Here's how the part is built. I have some questions about the finished solid (model axes, mm). A direction names the side the tool comes from. Round coordinates to 2 decimals unless told otherwise and drop trailing zeros. Loops run counter-clockwise (first coordinate to the right, second up) from the corner with the lowest first, then second, coordinate; pieces in that order, holes last. Notation, with made-up numbers: M 9,50 L 14,50 A29 ccw 14,88 Z; hole C 11.25,-22 d6. An arc over 180 degrees is marked long. Use a Markdown table: item, result.
from build123d import *

# Parameters (mm, degrees)
SKETCH1_W                    = 112.686822752
SKETCH1_H                    = 63.120861651
SKETCH1_R                    = 5.443424695
BASE_FLANGE1_DEPTH           = 0.7366
EDGE_FLANGE1_STRIP_W         = 4.4196
EDGE_FLANGE1_STRIP_H         = 0.7366
EDGE_FLANGE1_STRIP_CUT_DEPTH = 112.686822752
EDGE_FLANGE1_DEPTH           = 112.686822752
EDGE_FLANGE2_STRIP_W         = 4.4196
EDGE_FLANGE2_STRIP_H         = 0.7366
EDGE_FLANGE2_STRIP_CUT_DEPTH = 112.686822752
EDGE_FLANGE2_DEPTH           = 112.686822752


# Sheet-metal steps are written as plain solids
with BuildPart() as part:
    # Sketch1 → Base-Flange1 (new body)
    with BuildSketch(Plane(origin=(0, 0, 0), x_dir=(1, 0, 0), z_dir=(0, 1, 0))):
        with Locations((56.343411376, 31.560430826)):
            Rectangle(SKETCH1_W, SKETCH1_H)
        with Locations(Location((50.380635498, 49.990828995, 0), (0, 0, 270))):
            Circle(SKETCH1_R, mode=Mode.SUBTRACT)
        with Locations(Location((50.380635498, 13.130032656, 0), (0, 0, 90))):
            Circle(SKETCH1_R, mode=Mode.SUBTRACT)
    extrude(amount=-BASE_FLANGE1_DEPTH)

    # Edge-Flange1 strip (across the edge) → Edge-Flange1 strip cut (cut)
    with BuildSketch(Plane(origin=(112.686822752, 0, -63.120861651), x_dir=(0, 0, 1), z_dir=(-1, 0, 0))):
        with Locations((-0.7366, -0.3683)):
            Rectangle(EDGE_FLANGE1_STRIP_W, EDGE_FLANGE1_STRIP_H)
    extrude(amount=EDGE_FLANGE1_STRIP_CUT_DEPTH, mode=Mode.SUBTRACT)

    # Edge-Flange1 section (across the edge) → Edge-Flange1 (add)
    with BuildSketch(Plane(origin=(112.686822752, 0, -63.120861651), x_dir=(0, 0, 1), z_dir=(-1, 0, 0))):
        with BuildLine():
            Line((0, 0.7366), (0, 3.2634))
            Line((0, 3.2634), (0.7366, 3.2634))
            Line((0.7366, 3.2634), (0.7366, 0.7366))
            ThreePointArc((0.7366, 0.7366), (0.952345145, 0.215745145), (1.4732, 0))
            Line((1.4732, 0), (1.4732, -0.7366))
            ThreePointArc((1.4732, -0.7366), (0.43149029, -0.30510971), (0, 0.7366))
        make_face()
    extrude(amount=EDGE_FLANGE1_DEPTH)

    # Edge-Flange2 strip (across the edge) → Edge-Flange2 strip cut (cut)
    with BuildSketch(Plane(origin=(112.686822752, 3.2634, -62.384261651), x_dir=(0, -1, 0), z_dir=(-1, 0, 0))):
        with Locations((-0.7366, -0.3683)):
            Rectangle(EDGE_FLANGE2_STRIP_W, EDGE_FLANGE2_STRIP_H)
    extrude(amount=EDGE_FLANGE2_STRIP_CUT_DEPTH, mode=Mode.SUBTRACT)

    # Edge-Flange2 section (across the edge) → Edge-Flange2 (add)
    with BuildSketch(Plane(origin=(112.686822752, 3.2634, -62.384261651), x_dir=(0, -1, 0), z_dir=(-1, 0, 0))):
        with BuildLine():
            Line((0, 0.7366), (0, 61.2634))
            Line((0, 61.2634), (0.7366, 61.2634))
            Line((0.7366, 61.2634), (0.7366, 0.7366))
            ThreePointArc((0.7366, 0.7366), (0.952345145, 0.215745145), (1.4732, 0))
            Line((1.4732, 0), (1.4732, -0.7366))
            ThreePointArc((1.4732, -0.7366), (0.43149029, -0.30510971), (0, 0.7366))
        make_face()
    extrude(amount=EDGE_FLANGE2_DEPTH)


solid = part.part
1. I need wall thicknesses on probe 1 along Y at (x, z) = (16, -15); probe 2 along X at (y, z) = (-0.4, -48); probe 3 along Z at (x, y) = (94.5, 3.05). Which ranges of each line are inside material? Lowest first, please. Write a range as from..to.
Answer sheet:
| item | result |
|---|---|
| probe 1 | -0.74..0, 2.53..3.26 |
| probe 2 | 0..45.31, 55.45..112.69 |
| probe 3 | -62.41..-1.12 |
2. We'd pull the mould along Z, two halves only. Please class faces 1 (the face through (57, 2.527, -31)), 2 (the face through (52.02, -0.36, -44.8)): +Z half, -Z half, draft (parallel to the pull), parting line (faces both ways), or undercut.
Answer sheet:
| item | result |
|---|---|
| face 1 | draft |
| face 2 | undercut |
3. Imagine slicing it at C-C, the plane z = -48.5. Write out the boundary of the cut face in (x, y).
Answer sheet:
| item | result |
|---|---|
| outline | M 0,-0.74 L 45.15,-0.74 L 45.15,0 L 0,0 Z; M 0,2.53 L 112.69,2.53 L 112.69,3.26 L 0,3.26 Z; M 55.62,-0.74 L 112.69,-0.74 L 112.69,0 L 55.62,0 Z |
4. Imagine slicing it at B-B, the plane x = 104. Write out the boundary of the cut face in (y, z), then the cut area to 3 significant figures.
Answer sheet:
| item | result |
|---|---|
| outline | M -0.74,-61.65 A1.47 ccw 0.74,-63.12 L 1.79,-63.12 A1.47 ccw 3.26,-61.65 L 3.26,-1.12 L 2.53,-1.12 L 2.53,-61.65 A0.74 cw 1.79,-62.38 L 0.74,-62.38 A0.74 cw 0,-61.65 L 0,0 L -0.74,0 Z |
| area | 93.3 mm2 |
5. For pin 1 Ø1.5 at (x, y) = (39, 2.5) entering from +Z; pin 2 Ø1.2 at (x, y) = (78, 1.5) entering from +Z; pin 3 Ø17.5 at (x, z) = (50.38, -13.13) entering from -Y, each with a flat end and sliding along its axis, tell me the tip position at first contact or that it passes through.
Answer sheet:
| item | result |
|---|---|
| pin 1 | z = -1.12 |
| pin 2 | z = -62.32 |
| pin 3 | y = -0.74 |
6. Which directions (+Z, -Z, +X, -X, +Y, -Y) give clear straight access to the entire face, cutting with the end or side of a thin tool? Please do faces 3 (the face through (0, 3, -31)), 4 (the face through (56, 0, -31)), 5 (the face through (46.7, -0.36, -9.12)).
Answer sheet:
| item | result |
|---|---|
| face 3 | +Z, -Z, -X, +Y, -Y |
| face 4 | +Z, +X, -X |
| face 5 | -Y |
7. Imagine slicing it at A-A, the plane z = -30. Write out the boundary of the cut face in (x, y).
Answer sheet:
| item | result |
|---|---|
| outline | M 0,-0.74 L 112.69,-0.74 L 112.69,0 L 0,0 Z; M 0,2.53 L 112.69,2.53 L 112.69,3.26 L 0,3.26 Z |
